from build123d import *

# Parameters (mm, degrees)
SKETCH1_W           = 21.93
SKETCH1_H           = 41.52
BOSS_EXTRUDE2_DEPTH = 11
SKETCH3_W           = 21.93
SKETCH3_H           = 8.38
SKETCH3_H_2         = 8.42274565
SKETCH3_H_3         = 8.694734819
SKETCH3_W_2         = 22
SKETCH3_H_4         = 8.022519531
CUT_EXTRUDE2_DEPTH  = 4.6
BOSS_EXTRUDE3_START = 20.76
SKETCH5_W           = 17.4
SKETCH5_H           = 6.25
BOSS_EXTRUDE3_DEPTH = 8.4
SKETCH6_R           = 2.15
CUT_EXTRUDE3_DEPTH  = 8.4
SKETCH7_W           = 17.4
SKETCH7_H           = 6.25
BOSS_EXTRUDE4_DEPTH = 8.4
SKETCH9_R           = 2.15
CUT_EXTRUDE4_DEPTH  = 6.25
FILLET2_R           = 0.5


with BuildPart() as part:
    # Sketch1 → Boss-Extrude2 (new body)
    with BuildSketch(Plane(origin=(0, 0, 0), x_dir=(1, 0, 0), z_dir=(0, 1, 0))):
        Rectangle(SKETCH1_W, SKETCH1_H)
    extrude(amount=BOSS_EXTRUDE2_DEPTH)

    # Sketch3 → Cut-Extrude2 (cut)
    with BuildSketch(Plane(origin=(0, 11, 0), x_dir=(1, 0, 0), z_dir=(0, 1, 0))):
        with Locations((0, -14.97)):
            Rectangle(SKETCH3_W, SKETCH3_H)
        with Locations((0, -4.968627175)):
            Rectangle(SKETCH3_W, SKETCH3_H_2)
        with Locations((0, 5.190113059)):
            Rectangle(SKETCH3_W, SKETCH3_H_3)
        with Locations((0.013958332, 15.148740234)):
            Rectangle(SKETCH3_W_2, SKETCH3_H_4)
    extrude(amount=-CUT_EXTRUDE2_DEPTH, mode=Mode.SUBTRACT)

    # Sketch5 → Boss-Extrude3 (add)
    with BuildSketch(Plane.XY.offset(BOSS_EXTRUDE3_START)):
        with Locations((0, 3.125184184)):
            Rectangle(SKETCH5_W, SKETCH5_H)
    extrude(amount=BOSS_EXTRUDE3_DEPTH)

    # Sketch6 → Cut-Extrude3 (cut)
    with BuildSketch(Plane(origin=(0, 6.250184184, 0), x_dir=(1, 0, 0), z_dir=(0, 1, 0))):
        with Locations((-3.9, -24.867133618)):
            Circle(SKETCH6_R)
        with Locations((3.9, -24.867133618)):
            Circle(SKETCH6_R)
    extrude(amount=-CUT_EXTRUDE3_DEPTH, mode=Mode.SUBTRACT)

    # Sketch7 → Boss-Extrude4 (add)
    with BuildSketch(Plane(origin=(0, 0, -20.76), x_dir=(-1, 0, 0), z_dir=(0, 0, -1))):
        with Locations((0, 3.128849309)):
            Rectangle(SKETCH7_W, SKETCH7_H)
    extrude(amount=BOSS_EXTRUDE4_DEPTH)

    # Sketch9 → Cut-Extrude4 (cut)
    with BuildSketch(Plane(origin=(0, 6.253849309, 0), x_dir=(1, 0, 0), z_dir=(0, 1, 0))):
        with Locations((-3.9, 25.32626204)):
            Circle(SKETCH9_R)
        with Locations((3.9, 25.32626204)):
            Circle(SKETCH9_R)
    extrude(amount=-CUT_EXTRUDE4_DEPTH, mode=Mode.SUBTRACT)

    # Fillet2
    fillet2_edges = [part.edges().sort_by_distance(p)[0] for p in [
        (8.7, 3.128849309, -29.16),
        (-8.7, 3.128849309, -29.16),
        (-10.965, 8.7, 19.16),
        (-10.965, 8.7, 10.78),
        (10.965, 8.7, 10.78),
        (10.965, 8.7, 19.16),
        (-10.965, 8.7, 9.18),
        (-10.965, 8.7, 0.75725435),
        (10.965, 8.7, 0.75725435),
        (10.965, 8.7, 9.18),
        (-10.965, 8.7, -0.84274565),
        (-10.965, 8.7, -9.537480469),
        (10.965, 8.7, -9.537480469),
        (10.965, 8.7, -0.84274565),
        (10.965, 8.7, -19.16),
        (-10.965, 8.7, -19.16),
        (10.965, 8.7, -11.137480469),
        (-10.965, 8.7, -11.137480469),
        (10.965, 5.5, 20.76),
        (10.965, 5.5, -20.76),
        (-10.965, 5.5, -20.76),
        (-10.965, 5.5, 20.76),
        (-8.7, 3.125184184, 29.16),
        (8.7, 3.125184184, 29.16),
    ]]
    fillet(fillet2_edges, radius=FILLET2_R)


solid = part.part
Geometry check sheet. Reference: the model listing, model coordinates, mm. A direction names the side the tool comes from. Round coordinates to 2 decimals unless told otherwise and drop trailing zeros. Order: outer loops, then holes, each group sorted by start corner. A loop starts at its lowest first (then second) coordinate and runs counter-clockwise, first axis right, second up. Notation, with made-up numbers: (8.25, 7.5) -> (26.25, 7.5) arc R27 cw to (26.25, 34.5) -> close; hole circle Ø4 at (4, -12). An arc over 180 degrees is marked (long way). Use one line per item in the form item = value.
1. Set-up check for faces 4 (the face through (0, 9, -9.537)), 5 (the face through (8.7, 3, 25)), 6 (the face through (0, 11, -20)): record each of +Z, -Z, +X, -X, +Y, -Y from which the full face is reachable in a straight line by a thin tool's end or side.
Working result:
face_4 = +X, -X, +Y
face_5 = +Z, +X, +Y, -Y
face_6 = +Z, -Z, +X, -X, +Y
2. Scan lines: line 1 along Z through (x, y) = (3.9, 3.5); line 2 along Z through (x, y) = (9.75, 9.75); line 3 along Y through (x, z) = (8, -13). Record each from-to range of solid material in increasing order. Write a range as from..to.
Working result:
line_1 = -29.16..-27.48, -23.18..22.72, 27.02..29.16
line_2 = -20.76..-19.16, -11.14..-9.54, -0.84..0.76, 9.18..10.78, 19.16..20.76
line_3 = 0..6.4
3. Cross-section at C-C, the plane z = -4. Enter the section's corners in (x, y) (3 decimals).
Working result:
outline = (-10.965, 0) -> (10.965, 0) -> (10.965, 6.4) -> (-10.965, 6.4) -> close
4. Mould release check, pull along X, two halves, no side actions. Record for faces 1 (the face through (0, 0, 0)), 2 (the face through (3.434, 3.169, 26.966)), 3 (the face through (-10.965, 3, 0)): pulls with the +X half, pulls with the -X half, needs draft (parallel to the pull), parting line crosses it, or undercut.
Working result:
face_1 = needs draft
face_2 = undercut
face_3 = pulls with the -X half
5. Cross-section at B-B, the plane y = 7. Count the separate pieces of the cut face and the enclosed holes in it, plus the area to 3 significant figures.
Working result:
separate_pieces = 5
enclosed_holes = 0
area = 174 mm^2
6. Go/stop test with flat-tipped pins: pin 1 (6.5 mm diameter, centred on x = -3, z = -23.5, fed in from +Y); pin 2 (3 mm diameter, centred on x = 5, z = -4.5, fed in from +Y); pin 3 (3 mm diameter, centred on x = 3, y = 9, fed in from -Z); pin 4 (7 mm diameter, centred on x = 3.9, z = -25.33, fed in from +Y). Record where each tip stops, or that it passes through.
Working result:
pin_1 = 11
pin_2 = 6.4
pin_3 = -20.76
pin_4 = 6.25
